The listing builds one solid part. Answer for the finished solid, in the listing's coordinates (mm). Face numbers are marked on the shaded views. A direction names the side the tool comes from. Coordinates: 2 decimals unless noted, no trailing zeros. Order: outer loops, then holes, each group sorted by start corner. A loop starts at its lowest first (then second) coordinate and runs counter-clockwise, first axis right, second up. Notation, with made-up numbers: (-37, 0) -> (-3, 0) arc R21 cw to (-3, 35) -> close; hole circle Ø5 at (77.25, 35.5). An arc over 180 degrees is marked (long way). Return JSON: item names as keys, results as strings.
Autodesk Inventor part; units mm, degrees
ref_plane "YZ Plane" through (0, 0, 0) normal (1, 0, 0) x (0, 1, 0)
ref_plane "XZ Plane" through (0, 0, 0) normal (0, 1, 0) x (-1, 0, 0)
ref_plane "XY Plane" through (0, 0, 0) normal (0, 0, 1) x (1, 0, 0)
ref_plane "작업 평면1" through (0, 0, -34) normal (0, 0, -1) x (-1, 0, 0)
sketch "스케치1" plane through (0, 0, -34) normal (0, 0, -1) x (-1, 0, 0)
  circle A0 centre (17.3, -18) radius 1.35
  line L0 (20.1, -44.6) -> (20.1, 8.5)
  line L1 (14.5, -42) -> (14.5, 11.5)
  circle A1 centre (17.3, 4) radius 1.35
  circle A2 centre (17.3, -18) radius 1.45
  circle A3 centre (17.3, 4) radius 1.45
  line L2 (14.7, -42) -> (14.7, 11.5)
  line L3 (14.7, 11.5) -> (20.1, 8.5)
  line L4 (14.7, -20.9546) -> (32.7, -20.9546)
  line L5 (32.7, -20.9546) -> (32.7, 8.5)
  line L6 (32.7, 8.5) -> (20.1, 8.5)
  line L7 (32.7, -20.9546) -> (26.7, -20.9546)
  line L8 (26.7, -20.9546) -> (26.7, 8.5)
  line L9 (26.7, 8.5) -> (32.7, 8.5)
  line L10 (32.7, 8.5) -> (32.7, -20.9546)
  line L11 (20.1, 8.5) -> (14.7, 8.5)
  point P0 (0, 0)
  dimension "d0" = 0.1
  dimension "d1" = 0.1
  dimension "d2" = 0.2
  dimension "d3" = 18
  dimension "d8" = 6
extrude "돌출1" add sketch "스케치1" along normal blind 3 contours L4 L2 L11 L0 | L0 L6 L8 L4 | L8 L6 L5 L4 | A2 | A3
sketch "스케치2" plane through (0, 0, -34) normal (0, 0, 1) x (1, 0, 0)
  line L0 (-20.1, 8.5) -> (-14.7, 11.5)
  line L1 (-14.7, 8.5) -> (-14.7, -20.9546)
  line L2 (-20.1, -44.6) -> (-20.1, 8.5)
  line L3 (-32.7, 8.5) -> (-14.7, 8.5)
  line L4 (-32.7, -20.9546) -> (-32.7, 8.5)
  line L5 (-14.7, -20.9546) -> (-32.7, -20.9546)
  line L6 (-20.1, -20.9546) -> (-32.7, -20.9546)
  line L7 (-32.7, -20.9546) -> (-32.7, 8.5)
  line L8 (-32.7, 8.5) -> (-20.1, 8.5)
  line L9 (-20.1, 8.5) -> (-20.1, -20.9546)
  line L10 (-20.1, -20.9546) -> (-14.7, -20.9546)
  line L11 (-14.7, 11.5) -> (-20.1, 8.5)
  circle A0 centre (-17.3, -18) radius 1.45
  circle A1 centre (-17.3, 4) radius 1.35
  circle A2 centre (-17.3, 4) radius 1.45
  circle A3 centre (-17.3, 4) radius 1.45
  circle A4 centre (-17.3, -18) radius 1.45
  point P0 (0, 0)
ref_plane "작업 평면2" through (0, 0, 0) normal (0, 0, 1) x (1, 0, 0)
sketch "스케치3" plane through (0, 0, 0) normal (0, 0, 1) x (1, 0, 0)
  line L0 (-32.7, 8.5) -> (-14.7, 8.5)
  line L1 (-32.7, -20.9546) -> (-32.7, 8.5)
  line L2 (-14.7, -20.9546) -> (-32.7, -20.9546)
  line L3 (-14.7, 8.5) -> (-14.7, -20.9546)
  line L4 (-20.1, -20.9546) -> (-32.7, -20.9546)
  line L5 (-32.7, -20.9546) -> (-32.7, 8.5)
  line L6 (-32.7, 8.5) -> (-20.1, 8.5)
  line L7 (-20.1, 8.5) -> (-20.1, -20.9546)
  line L8 (-32.7, -20.9546) -> (-20.1, -20.9546)
  line L9 (-20.1, -20.9546) -> (-20.1, 8.5)
  line L10 (-20.1, 8.5) -> (-32.7, 8.5)
  line L11 (-32.7, 8.5) -> (-32.7, -20.9546)
  line L12 (-20.1, -20.9546) -> (-14.7, -20.9546)
  line L13 (-14.7, 8.5) -> (-14.7, -20.9546)
  line L14 (-14.7, 11.5) -> (-20.1, 8.5)
  circle A0 centre (-17.3, -18) radius 1.45
  circle A1 centre (-17.3, 4) radius 1.45
  circle A2 centre (-17.3, 4) radius 1.35
  circle A3 centre (-17.3, -18) radius 1.35
  point P0 (0, 0)
  dimension "d26" = 2.7
  dimension "d27" = 2.7
extrude "돌출2" add sketch "스케치3" along normal blind 3 contours L0 L7 L2 L1 | L0 L3 L2 L7 | A0 | A1
sketch "스케치4" plane through (0, 0, -34) normal (0, 0, 1) x (1, 0, 0)
  line L0 (-14.7, -20.9546) -> (-14.7, 8.5)
  line L1 (-14.7, 8.5) -> (-32.7, 8.5)
  line L2 (-32.7, 8.5) -> (-32.7, -20.9546)
  line L3 (-32.7, -20.9546) -> (-14.7, -20.9546)
  line L4 (-32.7, 8.5) -> (-26.7, 8.5)
  line L5 (-26.7, -20.9546) -> (-32.7, -20.9546)
  line L6 (-32.7, -20.9546) -> (-32.7, 8.5)
  line L7 (-32.7, 8.5) -> (-29.7, 8.5)
  line L8 (-29.7, 8.5) -> (-29.7, -20.9546)
  line L9 (-29.7, -20.9546) -> (-32.7, -20.9546)
  line L10 (-32.7, -20.9546) -> (-32.7, 8.5)
  point P0 (0, 0)
  point P1 (-29.7, -20.9546)
extrude "돌출3" add sketch "스케치4" along normal up to surface (34 mm away) contours L3 L2 L1 L8
sketch "스케치5" plane through (-32.7, -20.9546, -37) normal (-1, 0, 0) x (0, 0, 1)
  line L0 (40, 29.4546) -> (0, 29.4546)
  line L1 (0, 0) -> (0, 29.4546)
  line L2 (40, 0) -> (0, 0)
  line L3 (40, 29.4546) -> (40, 0)
  line L4 (40, 0) -> (0, 0)
  circle A0 centre (20, 14.7273) radius 14
  arc A1 (15, 20.2502) -> (25, 20.2502) centre (20, 14.7273) ccw
  circle A2 centre (20, 14.7273) radius 1.6
  circle A3 centre (12.2218, 22.5055) radius 1.35
  circle A4 centre (27.7782, 22.5055) radius 1.35
  circle A5 centre (27.7782, 6.9491) radius 1.35
  circle A6 centre (12.2218, 6.9491) radius 1.35
  arc A7 (15.6711, 19.5089) -> (24.3289, 19.5089) centre (20, 14.7273) ccw
  circle A8 centre (20, 14.7273) radius 6.45
  point P0 (37, 20.9546)
  point P1 (24.3289, 19.5089)
  point P2 (15.6711, 19.5089)
  dimension "d20" = 3.2
  dimension "d21" = 2.7
  dimension "d22" = 2.7
  dimension "d23" = 2.7
  dimension "d24" = 2.7
  dimension "d25" = 1
extrude "돌출4" cut sketch "스케치5" against normal blind 10 contours A2 | A3 | A4 | A5 | A6 | A8 A7
fillet "모깎기1" radius 1 4 edges at (-32.7, -6.2273, 3) (-32.7, -6.2273, -37) (-29.7, -6.2273, -34) (-29.7, -6.2273, 0)
properties part number "3D_ankle2" material "PMMA 플라스틱"
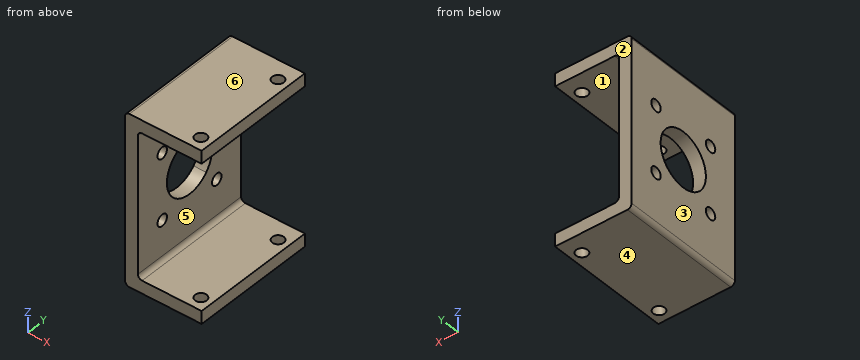
1. Determine the mould class of the marked faces 3, 4, 5 and 6 for opening direction Z: pulls with the +Z half, pulls with the -Z half, needs draft (parallel to the pull), parting line crosses it, or undercut.
Answer block:
{"face 3": "needs draft", "face 4": "pulls with the -Z half", "face 5": "undercut", "face 6": "pulls with the +Z half"}
2. For the marked faces 1 and 2, determine the directions among +Z, -Z, +X, -X, +Y, -Y from which every point of the face is accessible in a straight line to the end or side of a thin tool.
Answer block:
{"face 1": "+X, +Y, -Y", "face 2": "+Z, -Z, +X, -X, +Y"}
3. Each of these flat-tipped pins is pushed along its axis until it touches: pin 1 Ø9 at (y, z) = (-4, -17.5) entering from +X; pin 2 Ø2.5 at (x, y) = (-17.3, -18) entering from -Z. Where does it stop, or does it pass through?
Answer block:
{"pin 1": "stops at x = -29.7", "pin 2": "passes through"}
4. The part is cut by section D-D on x = -28.25. Give the vertices of the cut face in (y, z).
Answer block:
{"outline": "(-20.95, -37) -> (8.5, -37) -> (8.5, -34) -> (-20.95, -34) -> close; (-20.95, 0) -> (8.5, 0) -> (8.5, 3) -> (-20.95, 3) -> close"}
5. The part is cut by section A-A on z = -17. Give the vertices of the cut face in (x, y), and give its area (3 significant figures).
Answer block:
{"outline": "(-32.7, -20.95) -> (-29.7, -20.95) -> (-29.7, -12.68) -> (-32.7, -12.68) -> close; (-32.7, 0.22) -> (-29.7, 0.22) -> (-29.7, 8.5) -> (-32.7, 8.5) -> close", "area": "49.7 mm2"}
6. The part is cut by section B-B on y = 4. Give the vertices of the cut face in (x, z), and give its area (3 significant figures).
Answer block:
{"outline": "(-32.7, -36) arc R1 ccw to (-31.7, -37) -> (-18.65, -37) -> (-18.65, -34) -> (-28.7, -34) arc R1 cw to (-29.7, -33) -> (-29.7, -1) arc R1 cw to (-28.7, 0) -> (-18.65, 0) -> (-18.65, 3) -> (-31.7, 3) arc R1 ccw to (-32.7, 2) -> close; (-15.95, -37) -> (-14.7, -37) -> (-14.7, -34) -> (-15.95, -34) -> close; (-15.95, 0) -> (-14.7, 0) -> (-14.7, 3) -> (-15.95, 3) -> close", "area": "194 mm2"}
7. Consider line 1 (Y direction, x = -17.3, z = -36.3); line 2 (Z direction, x = -23.25, y = 6.75); line 3 (X direction, y = -18.75, z = -30). Determine where each line is inside the solid, lowest interval first. Write a range as from..to.
Answer block:
{"line 1": "y = -20.95..-19.35, -16.65..2.65, 5.35..8.5", "line 2": "z = -37..-34, 0..3", "line 3": "x = -32.7..-29.7"}
8. The part is cut by section C-C on x = -17.3. Give the vertices of the cut face in (y, z).
Answer block:
{"outline": "(-20.95, -37) -> (-19.35, -37) -> (-19.35, -34) -> (-20.95, -34) -> close; (-20.95, 0) -> (-19.35, 0) -> (-19.35, 3) -> (-20.95, 3) -> close; (-16.65, -37) -> (2.65, -37) -> (2.65, -34) -> (-16.65, -34) -> close; (-16.65, 0) -> (2.65, 0) -> (2.65, 3) -> (-16.65, 3) -> close; (5.35, -37) -> (8.5, -37) -> (8.5, -34) -> (5.35, -34) -> close; (5.35, 0) -> (8.5, 0) -> (8.5, 3) -> (5.35, 3) -> close"}
